```python
from build123d import *

# Parameters (mm, degrees)
SKETCH_1_W                       = 55
SKETCH_1_H                       = 55
SKETCH_1_R                       = 13
SKETCH_1_R_2                     = 2
SM_BASE_FLANGE_1_DEPTH           = 2
SM_EDGE_FLANGE_1_STRIP_W         = 9.4732
SM_EDGE_FLANGE_1_STRIP_H         = 2
SM_EDGE_FLANGE_1_STRIP_CUT_DEPTH = 55
SM_EDGE_FLANGE_1_DEPTH           = 55
SKETCH_9_R                       = 15
SKETCH_9_R_2                     = 2.5
CUT_EXTRUDE_1_DEPTH              = 10
EXTRUDE_1_DEPTH                  = 2
EXTRUDE_2_DEPTH                  = 2


# Sheet-metal steps are written as plain solids
with BuildPart() as part:
    # Sketch 1 → 基体-法兰1 (new body)
    with BuildSketch(Plane(origin=(0, 0, 0), x_dir=(1, 0, 0), z_dir=(0, 1, 0))):
        with Locations((0, -2)):
            Rectangle(SKETCH_1_W, SKETCH_1_H)
        with Locations(Location((0, 0, 0), (0, 0, 270))):
            Circle(SKETCH_1_R, mode=Mode.SUBTRACT)
        with Locations(Location((17.5, 0, 0), (0, 0, 270))):
            Circle(SKETCH_1_R_2, mode=Mode.SUBTRACT)
        with Locations(Location((-17.5, 0, 0), (0, 0, 270))):
            Circle(SKETCH_1_R_2, mode=Mode.SUBTRACT)
        with Locations(Location((0, 17.5, 0), (0, 0, 270))):
            Circle(SKETCH_1_R_2, mode=Mode.SUBTRACT)
        with Locations(Location((0, -17.5, 0), (0, 0, 270))):
            Circle(SKETCH_1_R_2, mode=Mode.SUBTRACT)
    extrude(amount=-SM_BASE_FLANGE_1_DEPTH)

    # 边线-法兰1 strip (across the edge) → 边线-法兰1 strip cut (cut)
    with BuildSketch(Plane(origin=(-27.5, 0, 29.5), x_dir=(0, 0, -1), z_dir=(1, 0, 0))):
        with Locations((-4, -1)):
            Rectangle(SM_EDGE_FLANGE_1_STRIP_W, SM_EDGE_FLANGE_1_STRIP_H)
    extrude(amount=SM_EDGE_FLANGE_1_STRIP_CUT_DEPTH, mode=Mode.SUBTRACT)

    # 边线-法兰1 section (across the edge) → 边线-法兰1 (add)
    with BuildSketch(Plane(origin=(-27.5, 0, 29.5), x_dir=(0, 0, -1), z_dir=(1, 0, 0))):
        with BuildLine():
            Line((-2, 0.7366), (-2, 58))
            Line((-2, 58), (0, 58))
            Line((0, 58), (0, 0.7366))
            ThreePointArc((0, 0.7366), (0.215745145, 0.215745145), (0.7366, 0))
            Line((0.7366, 0), (0.7366, -2))
            ThreePointArc((0.7366, -2), (-1.198468417, -1.198468417), (-2, 0.7366))
        make_face()
    extrude(amount=SM_EDGE_FLANGE_1_DEPTH)

    # 草图9 → 切除-拉伸1 (cut)
    with BuildSketch(Plane(origin=(0, 0, 29.5), x_dir=(-1, 0, 0), z_dir=(0, 0, -1))):
        with Locations((0, 30.7366)):
            Circle(SKETCH_9_R)
        with Locations((-15, 45.7366)):
            Circle(SKETCH_9_R_2)
        with Locations((-15, 15.7366)):
            Circle(SKETCH_9_R_2)
        with Locations((15, 15.7366)):
            Circle(SKETCH_9_R_2)
        with Locations((15, 45.7366)):
            Circle(SKETCH_9_R_2)
    extrude(amount=-CUT_EXTRUDE_1_DEPTH, mode=Mode.SUBTRACT)

    # 草图10 → 凸台-拉伸1 (add)
    with BuildSketch(Plane(origin=(27.5, 0, 0), x_dir=(0, 0, -1), z_dir=(1, 0, 0))):
        Polygon((-29.5, 29.3683), (0, 0), (-29.5, 0), align=None)
    extrude(amount=-EXTRUDE_1_DEPTH)

    # 草图11 → 凸台-拉伸2 (add)
    with BuildSketch(Plane.ZY.offset(27.5)):
        Polygon((29.5, 29.3683), (0, 0), (29.5, 0), align=None)
    extrude(amount=-EXTRUDE_2_DEPTH)


solid = part.part
```
Part model, mm, in its own coordinate system. A direction names the side the tool comes from. Round coordinates to 2 decimals unless told otherwise and drop trailing zeros. Loops run counter-clockwise (first coordinate to the right, second up) from the corner with the lowest first, then second, coordinate; pieces in that order, holes last. Notation, with made-up numbers: (27, -40) -> (64, -40) arc R12 cw to (64, -27) -> close; hole circle Ø9 at (85, 67.5). An arc over 180 degrees is marked (long way). Use CSV: the item, a comma, the result in double quotes. Start each with the question number.
1) Cut at B-B, the plane x = 0. Write the cut outline in (y, z).
2) Cut at D-D, the plane x = 8. Write the cut outline in (y, z).
3) Cut at A-A, the plane z = -17.5. Write the cut outline in (x, y).
4) Which spindle directions (+Z, -Z, +X, -X, +Y, -Y) get a long thin tool onto all of the face, cutting with end or side? Do faces 4 (the flat face through (0, -1, -25.5)), 5 (the flat face through (-0.4, 0, 13.3)). Say none if no direction does.
5) Drop flat-ended pins along their axis: P1, Ø3.5, axis at x = -17.5, z = 0, coming from the -Y side; P2, Ø6, axis at x = 12, z = -17, coming from the +Y side; P3, Ø4, axis at x = -0.5, y = 45.5, coming from the -Z side. Give the stop position or say it passes through.
6) Wall check: L1, parallel to X at y = 3, z = 28; L2, parallel to Z at x = 8.5, y = 47; L3, parallel to Y at x = 22, z = 10. Give the ranges that are in metal, low to high. Write a range as [from, to].
7) Pull direction Z, two halves, no side cores. Call faces 1 (the flat face through (-6.5, 17, 29.5)), 2 (the cylindrical face through (-13.016, 14.215, 30.486)), 3 (the cylindrical face through (19.483, -0.986, -0.26)): +Z half, -Z half, draft (parallel to the pull), parting line (faces both ways), or undercut.
8) Cut at C-C, the plane y = 24. Write the cut outline in (x, z).
Determined:
1,outline,"(-2, -25.5) -> (0, -25.5) -> (0, -19.5) -> (-2, -19.5) -> close; (-2, -15.5) -> (0, -15.5) -> (0, -13) -> (-2, -13) -> close; (-2, 13) -> (0, 13) -> (0, 15.5) -> (-2, 15.5) -> close; (-2, 19.5) -> (0, 19.5) -> (0, 28.76) arc R0.74 cw to (0.74, 29.5) -> (15.74, 29.5) -> (15.74, 31.5) -> (0.74, 31.5) arc R2.74 ccw to (-2, 28.76) -> close; (45.74, 29.5) -> (58, 29.5) -> (58, 31.5) -> (45.74, 31.5) -> close"
2,outline,"(-2, -25.5) -> (0, -25.5) -> (0, -10.25) -> (-2, -10.25) -> close; (-2, 10.25) -> (0, 10.25) -> (0, 28.76) arc R0.74 cw to (0.74, 29.5) -> (18.05, 29.5) -> (18.05, 31.5) -> (0.74, 31.5) arc R2.74 ccw to (-2, 28.76) -> close; (43.43, 29.5) -> (58, 29.5) -> (58, 31.5) -> (43.43, 31.5) -> close"
3,outline,"(-27.5, -2) -> (-2, -2) -> (-2, 0) -> (-27.5, 0) -> close; (2, -2) -> (27.5, -2) -> (27.5, 0) -> (2, 0) -> close"
4,face 4,"-Z, +X, -X, +Y, -Y"
4,face 5,"-Z, +Y"
5,P1,"passes through"
5,P2,"stops at y = 0"
5,P3,"stops at z = 29.5"
6,L1,"x = [-27.5, -25.5], [25.5, 27.5]"
6,L2,"z = [29.5, 31.5]"
6,L3,"y = [-2, 0]"
7,face 1,"-Z half"
7,face 2,"draft"
7,face 3,"undercut"
8,outline,"(-27.5, 24.11) -> (-25.5, 24.11) -> (-25.5, 29.5) -> (-13.4, 29.5) -> (-13.4, 31.5) -> (-27.5, 31.5) -> close; (13.4, 29.5) -> (25.5, 29.5) -> (25.5, 24.11) -> (27.5, 24.11) -> (27.5, 31.5) -> (13.4, 31.5) -> close"
